Geometry check sheet. Reference: the model listing, model coordinates, mm. A direction names the side the tool comes from. Give positions to 0.01 mm unless a question says otherwise; leave off trailing zeros. Loops run counter-clockwise (first coordinate to the right, second up) from the corner with the lowest first, then second, coordinate; pieces in that order, holes last.
1. Material ranges on L1, parallel to Y at x = 7.75, z = 24.5; L2, parallel to Z at x = 5.5, y = -7.5; L3, parallel to Y at x = 12, z = 36.5, recorded low to high.
2. Cross-section at D-D, the plane z = 14. Record the cut outline in (x, y) (3 decimals), plus the area to 3 significant figures.
3. Release check for a two-part mould opening along Z. For faces 1 (the cylindrical face through (14, -27, 22)), 2 (the flat face through (0, -12, -20)), 3 (the cylindrical face through (11.268, -23.395, -17.834)) record: +Z half, -Z half, draft (parallel to the pull), parting line (faces both ways), or undercut.
4. Go/stop test with flat-tipped pins: pin 1 Ø2 at (x, y) = (4.5, 9.5) entering from +Z; pin 2 Ø11 at (x, z) = (8.5, 11) entering from +Y; pin 3 Ø8 at (y, z) = (1, -12) entering from -X; pin 4 Ø7.5 at (x, z) = (11.11, 20.48) entering from -Y. Record where each tip stops, or that it passes through.
5. Cross-section at A-A, the plane z = 20.5. Record the cut outline in (x, y) (3 decimals).
6. Tool access check on faces 4 (the flat face through (11, -24.831, 10)), 5 (the cylindrical face through (12.09, -7.44, -21.55)). Record the directions out of +Z, -Z, +X, -X, +Y, -Y that give a thin tool (end or side, any length) a straight path to the whole face; none if there is none.
7. Cross-section at C-C, the plane x = 18.25. Record the cut outline in (y, z).
8. Cross-section at B-B, the plane x = 9.75. Record the cut outline in (y, z), plus the area to 3 significant figures.
from build123d import *

# Parameters (mm, degrees)
EXTRUDE1_DEPTH     = 22.225
SKETCH2_R          = 3.2639
CUT_EXTRUDE1_DEPTH = 22.225
FILLET1_R          = 4.7752


with BuildPart() as part:
    # Sketch1 → Extrude1 (new body)
    with BuildSketch(Plane(origin=(0, 0, 0), x_dir=(0, 0, -1), z_dir=(1, 0, 0))):
        with BuildLine():
            Line((23.97075862, -29.606090317), (19.19555862, -24.830890317))
            Line((19.19555862, -24.830890317), (-34.75404138, -24.830890317))
            ThreePointArc((-34.75404138, -24.830890317), (-38.130617682, -26.229514015), (-39.52924138, -29.606090317))
            Line((-39.52924138, -29.606090317), (23.97075862, -29.606090317))
        make_face()
    extrude(amount=EXTRUDE1_DEPTH)

    # Sketch2 → Cut-Extrude1 (cut)
    with BuildSketch(Plane(origin=(0, -24.830890317, 0), x_dir=(1, 0, 0), z_dir=(0, 1, 0))):
        with Locations(Location((11.1125, -20.47924138, 0), (0, 0, 270))):  # turned: the seam where the file's is
            Circle(SKETCH2_R)
        with Locations(Location((11.1125, 4.92075862, 0), (0, 0, 270))):  # turned: the seam where the file's is
            Circle(SKETCH2_R)
    extrude(amount=-CUT_EXTRUDE1_DEPTH, mode=Mode.SUBTRACT)

    # Mirror1: part across plane


with BuildPart() as part_1:
    add(part.part)
    add(part.part.mirror(Plane(origin=(22.225, -29.606090317, -23.97075862), x_dir=(0, 0.707106781, 0.707106781), z_dir=(0, -0.707106781, 0.707106781))))

    # Fillet1
    fillet1_edges = [part_1.edges().sort_by_distance(p)[0] for p in [
        (11.1125, -24.830890317, -19.19555862),
    ]]
    fillet(fillet1_edges, radius=FILLET1_R)


solid = part_1.part
Result:
1. L1: y = -29.61 to -24.83
1. L2: z = -23.97 to -19.2
1. L3: y = -29.61 to -25.16
2. outline: (0, -29.606) - (22.225, -29.606) - (22.225, -24.831) - (0, -24.831) - close
2. area: 106 mm2
3. face 1: undercut
3. face 2: draft
3. face 3: +Z half
4. pin 1: stops at z = -19.2
4. pin 2: stops at y = -24.83
4. pin 3: passes through
4. pin 4: stops at y = -29.61
5. outline: (0, -29.606) - (7.849, -29.606) - (7.849, -24.831) - (0, -24.831) - close; (14.376, -29.606) - (22.225, -29.606) - (22.225, -24.831) - (14.376, -24.831) - close
6. face 4: +Z, +X, -X, +Y
6. face 5: +Z, -Z
7. outline: (-29.61, -23.97) - (33.89, -23.97) arc R4.78 ccw to (29.12, -19.2) - (-20.06, -19.2) arc R4.78 cw to (-24.83, -14.42) - (-24.83, 34.75) arc R4.78 ccw to (-29.61, 39.53) - close
8. outline: (-29.61, -23.97) - (-13.52, -23.97) - (-13.52, -19.2) - (-20.06, -19.2) arc R4.78 cw to (-24.83, -14.42) - (-24.83, -7.89) - (-29.61, -7.89) - close; (-29.61, -1.95) - (-24.83, -1.95) - (-24.83, 17.51) - (-29.61, 17.51) - close; (-29.61, 23.45) - (-24.83, 23.45) - (-24.83, 34.75) arc R4.78 ccw to (-29.61, 39.53) - close; (-7.59, -23.97) - (11.88, -23.97) - (11.88, -19.2) - (-7.59, -19.2) - close; (17.81, -23.97) - (33.89, -23.97) arc R4.78 ccw to (29.12, -19.2) - (17.81, -19.2) - close
8. area: 465 mm2
